Here's the drawing with two shaded views (mm, measured from the low corner). I have some questions. A direction names the side the tool comes from. Round coordinates to 2 decimals unless told otherwise and drop trailing zeros. Loops run counter-clockwise (first coordinate to the right, second up) from the corner with the lowest first, then second, coordinate; pieces in that order, holes last. Notation, with made-up numbers: (65, -20.75) -> (86, -20.75) arc R15 cw to (86, 1.25) -> close; hole circle Ø1 at (16, 0.25). An arc over 180 degrees is marked (long way). Write each question's results on one line, items separated by ' | '. Start each with the question number.
1) For P1, Ø1.5, axis at y = 1.5, z = 22.5, coming from the -X side; P2, Ø3, axis at x = 15.5, z = 22.5, coming from the +Y side; P3, Ø1.6, axis at y = 5.5, z = 26.5, coming from the +X side, each with a flat end and sliding along its axis, tell me the tip position at first contact or that it passes through.
2) Imagine slicing it at A-A, the plane x = 12. List the corners of the cut face in (y, z) for me.
3) Imagine slicing it at D-D, the plane x = 2. List the corners of the cut face in (y, z) for me.
4) Imagine slicing it at B-B, the plane z = 20. List the corners of the cut face in (x, y) for me, plus the area to 3 significant figures.
5) Which directions (+Z, -Z, +X, -X, +Y, -Y) give clear straight access to the entire face, cutting with the end or side of a thin tool? Please do the marked faces 1 and 2.
6) If I drill on probe 1 along X at (y, z) = (2.75, 6.5); probe 2 along Y at (x, z) = (12.5, 55.5); probe 3 along X at (y, z) = (12, 22), over which ranges is the centre line in solid material (lowest first)?
7) Imagine slicing it at C-C, the plane y = 8. List the corners of the cut face in (x, z) for me (1 decimal), plus the area to 3 significant figures.
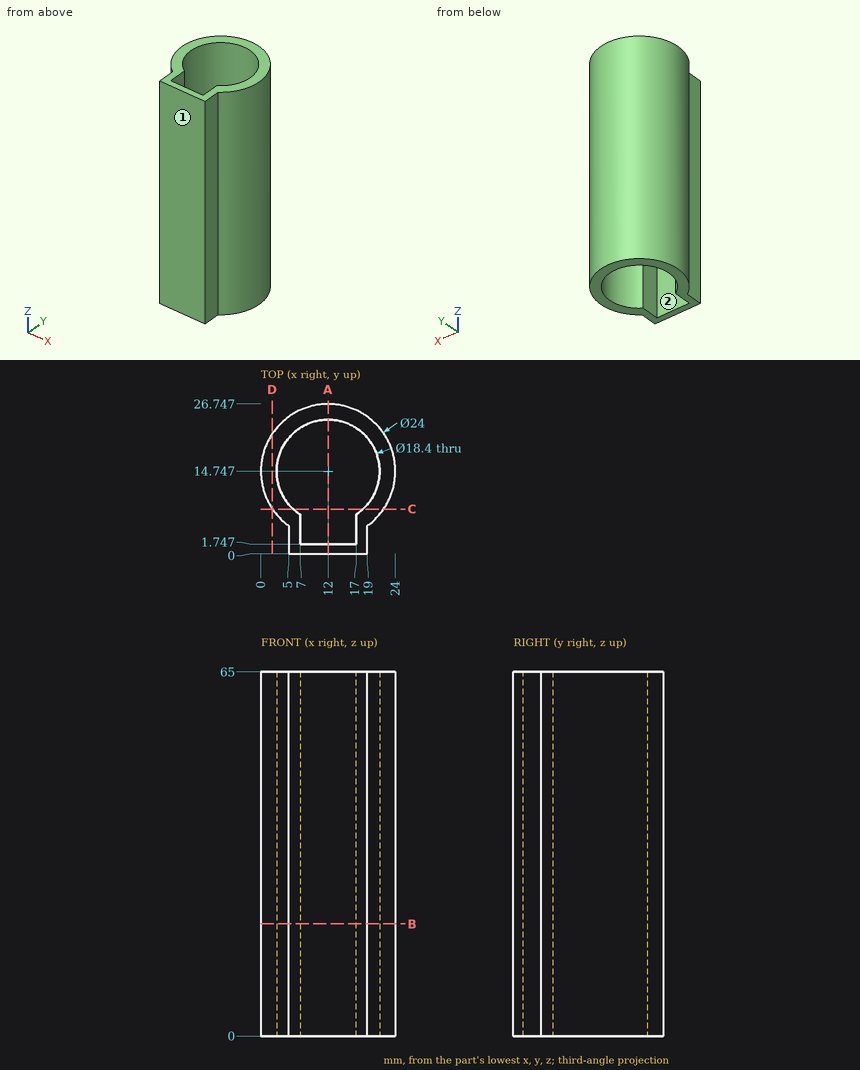
Checked values:
1) P1: x = 5 | P2: y = 26.58 | P3: x = 20.52
2) outline: (0, 0) -> (1.75, 0) -> (1.75, 65) -> (0, 65) -> close; (23.95, 0) -> (26.75, 0) -> (26.75, 65) -> (23.95, 65) -> close
3) outline: (8.11, 0) -> (21.38, 0) -> (21.38, 65) -> (8.11, 65) -> close
4) outline: (5, 0) -> (19, 0) -> (19, 5) arc R12 ccw (long way) to (5, 5) -> close; hole (7, 1.75) -> (17, 1.75) -> (17, 7.02) arc R9.2 ccw (long way) to (7, 7.02) -> close | area: 192 mm^2
5) face 1: +Z, -Z, +X, -X, -Y | face 2: +Z, -Z
6) probe 1: 5 to 7, 17 to 19 | probe 2: 0 to 1.75, 23.93 to 26.74 | probe 3: 0.32 to 3.22, 20.78 to 23.68
7) outline: (2.1, 0) -> (5.7, 0) -> (5.7, 65) -> (2.1, 65) -> close; (18.3, 0) -> (21.9, 0) -> (21.9, 65) -> (18.3, 65) -> close | area: 477 mm^2
